```python
from build123d import *

# Parameters (mm, degrees)
BOSS_EXTRUDE1_DEPTH = 40.1
SKETCH3_R           = 1.35
CUT_EXTRUDE2_DEPTH  = 50.8
SKETCH4_R           = 1.016
CUT_EXTRUDE3_DEPTH  = 50.8
SKETCH6_W           = 62.086073973
SKETCH6_H           = 34.1
CUT_EXTRUDE4_DEPTH  = 6
SKETCH17_W          = 33.483743456
SKETCH17_H          = 71.762692688
CUT_EXTRUDE5_DEPTH  = 101.73954578


with BuildPart() as part:
    # Sketch1 → Boss-Extrude1 (new body)
    with BuildSketch(Plane.XY):
        Polygon((0, 0), (0, 52.578), (6, 52.578), (6, 8.5), (76, 8.5), (76, 0), align=None)
    extrude(amount=BOSS_EXTRUDE1_DEPTH)

    # Sketch3 → Cut-Extrude2 (cut)
    with BuildSketch(Plane.XY.offset(40.1)):
        with Locations((27.996, 2.8)):
            Circle(SKETCH3_R)
        with Locations((49.996, 2.8)):
            Circle(SKETCH3_R)
        with Locations((71.996, 2.8)):
            Circle(SKETCH3_R)
    extrude(amount=-CUT_EXTRUDE2_DEPTH, mode=Mode.SUBTRACT)

    # Sketch4 → Cut-Extrude3 (cut)
    with BuildSketch(Plane.ZY):
        with Locations((27.88, 17.6)):
            Circle(SKETCH4_R)
        with Locations(Location((11.88, 17.6, 0), (0, 0, 270))):
            Circle(SKETCH4_R)
        with Locations((27.88, 49.6)):
            Circle(SKETCH4_R)
        with Locations(Location((11.88, 49.6, 0), (0, 0, 270))):
            Circle(SKETCH4_R)
    extrude(amount=-CUT_EXTRUDE3_DEPTH, mode=Mode.SUBTRACT)

    # Sketch6 → Cut-Extrude4 (cut)
    with BuildSketch(Plane.XZ):
        with Locations((50.043036987, 20.05)):
            Rectangle(SKETCH6_W, SKETCH6_H)
    extrude(amount=-CUT_EXTRUDE4_DEPTH, mode=Mode.SUBTRACT)

    # Sketch17 → Cut-Extrude5 (cut, through all)
    with BuildSketch(Plane.XY.offset(40.1)):
        with Locations((7.254128272, 35.881346344)):
            Rectangle(SKETCH17_W, SKETCH17_H)
    extrude(amount=-CUT_EXTRUDE5_DEPTH, mode=Mode.SUBTRACT)


solid = part.part
```
Design review of the part built by this model. Coordinates are the model's own, in mm. A direction names the side the tool comes from. Round coordinates to 2 decimals unless told otherwise and drop trailing zeros. Write each loop counter-clockwise with the first axis right and the second up, starting at its lowest first coordinate (ties: lowest second). Pieces come first, ordered by that corner, then holes. Notation, with made-up numbers: (87, -30.75) -> (104, -30.75) arc R11 ccw to (104, -18.75) -> close; hole circle Ø9 at (57.5, -35.5). An arc over 180 degrees is marked (long way). Answer in a Markdown table with one row per item.
Q1. To check wall thickness, follow L1, parallel to Z at x = 67.5, y = 3.25; L2, parallel to Y at x = 45, z = 23.5. State the ranges of each line that lie inside material, in increasing order. Write a range as [from, to].
The answers:
| item | result |
|---|---|
| L1 | [0, 3], [37.1, 40.1] |
| L2 | [6, 8.5] |
Q2. Clearance check with flat-ended pins moving along their axes: pin 1 Ø3.5 at (x, y) = (71.996, 2.8) entering from +Z; pin 2 Ø3 at (x, z) = (59.5, 19.5) entering from -Y. State where each tip first meets the part, or that it passes through.
The answers:
| item | result |
|---|---|
| pin 1 | z = 40.1 |
| pin 2 | y = 6 |
Q3. Take a section at D-D, the plane z = 34. State the section outline as (x, y) points.
The answers:
| item | result |
|---|---|
| outline | (24, 6) -> (76, 6) -> (76, 8.5) -> (24, 8.5) -> close |
Q4. Take a section at A-A, the plane y = 2.8. Count the separate pieces of the cut face and the enclosed holes in it, then the cut area to 3 significant figures.
The answers:
| item | result |
|---|---|
| separate pieces | 8 |
| enclosed holes | 0 |
| area | 263 mm² |
Q5. Draft analysis for pull direction Y (two halves, no side actions). For faces 3 (the face through (50, 8.5, 20)), 4 (the face through (50, 0, 39)), 5 (the face through (51.284, 3.206, 38.621)), 6 (the face through (23.996, 7, 20)), state which applies: +Y half, -Y half, draft (parallel to the pull), parting line (faces both ways), or undercut.
The answers:
| item | result |
|---|---|
| face 3 | +Y half |
| face 4 | -Y half |
| face 5 | undercut |
| face 6 | draft |
Q6. Take a section at B-B, the plane x = 49.5. State the section outline as (y, z) points, then the cut area to 3 significant figures.
The answers:
| item | result |
|---|---|
| outline | (0, 0) -> (1.54, 0) -> (1.54, 3) -> (0, 3) -> close; (0, 37.1) -> (1.54, 37.1) -> (1.54, 40.1) -> (0, 40.1) -> close; (4.06, 0) -> (8.5, 0) -> (8.5, 40.1) -> (4.06, 40.1) -> (4.06, 37.1) -> (6, 37.1) -> (6, 3) -> (4.06, 3) -> close |
| area | 121 mm² |
Q7. For faces 1 (the face through (49.6, 4.3, 3)), 2 (the face through (29.284, 3.206, 1.521)), list the 3-axis set-ups (+Z, -Z, +X, -X, +Y, -Y) from which the entire face can be reached by the end or side of a thin tool; tool diameter is ignored.
The answers:
| item | result |
|---|---|
| face 1 | +X, -X, -Y |
| face 2 | +Z, -Z |
Q8. Take a section at C-C, the plane x = 30.5. State the section outline as (y, z) points.
The answers:
| item | result |
|---|---|
| outline | (0, 0) -> (8.5, 0) -> (8.5, 40.1) -> (0, 40.1) -> (0, 37.1) -> (6, 37.1) -> (6, 3) -> (0, 3) -> close |
